Can you work these out from the model? Positions are in its coordinate system, mm. Face numbers are marked on the shaded views. A direction names the side the tool comes from. Round coordinates to 2 decimals unless told otherwise and drop trailing zeros. Loops run counter-clockwise (first coordinate to the right, second up) from the corner with the lowest first, then second, coordinate; pieces in that order, holes last.
(1) Will these pins go through, and if not, where does the flat tip stop? pin 1 Ø0.9 at (y, z) = (3.5, 1) entering from +X; pin 2 Ø0.9 at (x, z) = (-3, 2) entering from +Y; pin 3 Ø1.5 at (x, z) = (14, 1) entering from -Y.
(2) I want a section at B-B on z = 0.95. Write out the boundary of the cut face in (x, y).
(3) I want a section at A-A on y = -2.25. Write out the boundary of the cut face in (x, z).
(4) Which directions (+Z, -Z, +X, -X, +Y, -Y) give clear straight access to the entire face, cutting with the end or side of a thin tool? Please do the marked faces 1, 2 and 3.
(5) I want a section at C-C on x = 15. Write out the boundary of the cut face in (y, z).
(6) If I drill on line 1 along X through (y, z) = (3, 1.8); line 2 along Y through (x, z) = (-10.5, 1.3), over which ranges is the centre line in solid material (lowest first)?
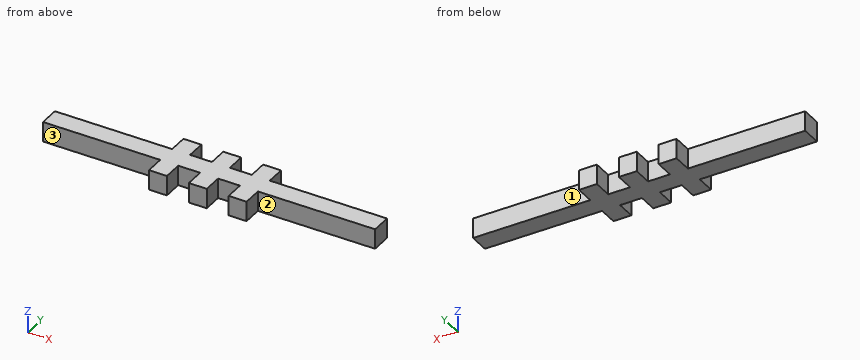
Autodesk Inventor part; units mm, degrees
ref_plane "YZ Plane" through (0, 0, 0) normal (1, 0, 0) x (0, 1, 0)
ref_plane "XZ Plane" through (0, 0, 0) normal (0, 1, 0) x (-1, 0, 0)
ref_plane "XY Plane" through (0, 0, 0) normal (0, 0, 1) x (1, 0, 0)
sketch "tabs" plane through (0, 0, 0) normal (0, 0, 1) x (1, 0, 0)
  line L0 (16.0425, 13.6368) -> (18.7425, 13.6368)
  line L1 (18.7425, 13.6368) -> (18.7425, 10.7868)
  line L2 (18.7425, 10.7868) -> (16.0425, 10.7868)
  line L3 (16.0425, 10.7868) -> (16.0425, 13.6368)
  line L4 (22.0425, 13.6368) -> (24.7425, 13.6368)
  line L5 (24.7425, 13.6368) -> (24.7425, 10.7868)
  line L6 (24.7425, 10.7868) -> (22.0425, 10.7868)
  line L7 (22.0425, 10.7868) -> (22.0425, 13.6368)
  line L8 (28.0425, 13.6368) -> (30.7425, 13.6368)
  line L9 (30.7425, 13.6368) -> (30.7425, 10.7868)
  line L10 (30.7425, 10.7868) -> (28.0425, 10.7868)
  line L11 (28.0425, 10.7868) -> (28.0425, 13.6368)
  line L12 (23.3925, 10.7868) -> (23.3925, 8.8536) construction
  point P0 (23.3925, 12.1901)
  dimension "d2" = 2.7
  dimension "d3" = 3.3
  dimension "d4" = 3.3
  dimension "d5" = 2.85
sketch "Sketch1" plane through (0, 0, 0) normal (0, 0, 1) x (1, 0, 0)
  line L0 (-25, 1.5) -> (25, 1.5)
  line L1 (25, 1.5) -> (25, -1.5)
  line L2 (25, -1.5) -> (-25, -1.5)
  line L3 (-25, -1.5) -> (-25, 1.5)
  line L4 (0, 16.9043) -> (0, -20.0235) construction
  line L5 (-32.3473, 0) -> (40.4078, 0) construction
  line L6 (-7.35, 4.35) -> (-4.65, 4.35)
  line L7 (-4.65, 4.35) -> (-4.65, 1.5)
  line L8 (-4.65, 1.5) -> (-7.35, 1.5)
  line L9 (-7.35, 1.5) -> (-7.35, 4.35)
  line L10 (-1.35, 4.35) -> (1.35, 4.35)
  line L11 (1.35, 4.35) -> (1.35, 1.5)
  line L12 (1.35, 1.5) -> (-1.35, 1.5)
  line L13 (-1.35, 1.5) -> (-1.35, 4.35)
  line L14 (4.65, 4.35) -> (7.35, 4.35)
  line L15 (7.35, 4.35) -> (7.35, 1.5)
  line L16 (7.35, 1.5) -> (4.65, 1.5)
  line L17 (4.65, 1.5) -> (4.65, 4.35)
  line L18 (0, 1.5) -> (0, -0.4332) construction
  line L19 (-7.35, -1.5) -> (-4.65, -1.5)
  line L20 (-4.65, -1.5) -> (-4.65, -4.35)
  line L21 (-4.65, -4.35) -> (-7.35, -4.35)
  line L22 (-7.35, -4.35) -> (-7.35, -1.5)
  line L23 (-1.35, -1.5) -> (1.35, -1.5)
  line L24 (1.35, -1.5) -> (1.35, -4.35)
  line L25 (1.35, -4.35) -> (-1.35, -4.35)
  line L26 (-1.35, -4.35) -> (-1.35, -1.5)
  line L27 (4.65, -1.5) -> (7.35, -1.5)
  line L28 (7.35, -1.5) -> (7.35, -4.35)
  line L29 (7.35, -4.35) -> (4.65, -4.35)
  line L30 (4.65, -4.35) -> (4.65, -1.5)
  line L31 (0, -4.35) -> (0, -6.2832) construction
  point P0 (0, 0)
  point P1 (0, 1.5)
  point P2 (25, 0)
  dimension "d0" = 50
  dimension "d1" = 3
extrude "Extrusion1" add sketch "Sketch1" along normal blind 3
equation "\"d2\" = mat + kerf"
equation "\"d3\" = mat - kerf"
equation "\"d4\" = mat - kerf"
equation "\"d5\" = mat + 0.5 * kerf"
equation "\"d1\" = mat"
equation "\"d6\" = mat"
properties part number "link1"
Filled sheet:
1. pin 1: stops at x = 7.35
1. pin 2: stops at y = 1.5
1. pin 3: stops at y = -1.5
2. outline: (-25, -1.5) - (-7.35, -1.5) - (-7.35, -4.35) - (-4.65, -4.35) - (-4.65, -1.5) - (-1.35, -1.5) - (-1.35, -4.35) - (1.35, -4.35) - (1.35, -1.5) - (4.65, -1.5) - (4.65, -4.35) - (7.35, -4.35) - (7.35, -1.5) - (25, -1.5) - (25, 1.5) - (7.35, 1.5) - (7.35, 4.35) - (4.65, 4.35) - (4.65, 1.5) - (1.35, 1.5) - (1.35, 4.35) - (-1.35, 4.35) - (-1.35, 1.5) - (-4.65, 1.5) - (-4.65, 4.35) - (-7.35, 4.35) - (-7.35, 1.5) - (-25, 1.5) - close
3. outline: (-7.35, 0) - (-4.65, 0) - (-4.65, 3) - (-7.35, 3) - close; (-1.35, 0) - (1.35, 0) - (1.35, 3) - (-1.35, 3) - close; (4.65, 0) - (7.35, 0) - (7.35, 3) - (4.65, 3) - close
4. face 1: +Z, -Z, +X, +Y
4. face 2: +Z, -Z, +X, -Y
4. face 3: +Z, -Z, -X, -Y
5. outline: (-1.5, 0) - (1.5, 0) - (1.5, 3) - (-1.5, 3) - close
6. line 1: x = -7.35 to -4.65, -1.35 to 1.35, 4.65 to 7.35
6. line 2: y = -1.5 to 1.5
